Geometry: see drawing. Coordinates: mm, zero at the bounding-box minimum. A direction names the side the tool comes from. Give positions to 0.01 mm unless a question says otherwise; leave off trailing zeros. Write each loop counter-clockwise with the first axis right and the second up, starting at its lowest first coordinate (ties: lowest second). Pieces come first, ordered by that corner, then holes. Notation, with made-up numbers: M 2,27.5 L 16,27.5 A19 cw 16,47.5 Z; hole C 89,29 d1. An arc over 180 degrees is marked long. Use a Markdown table: item, result. Add a question column.
(1) Cut plane B-B (y = 21). Output: boundary loops of the cut face in (x, z).
(2) Material intervals for L1, parallel to Z at x = 5, y = 17; L2, parallel to Y at x = 2.5, z = 15.5; L3, parallel to Z at x = 7, y = 7.5, sorted ascending.
(3) Draft query along Z for the marked faces 4, 5, 6 and 7. Return one class per face: released by +Z, released by -Z, zero draft, split by the parting line, or undercut.
(4) Cut plane A-A (z = 6). Output: boundary loops of the cut face in (x, y).
(5) Cut plane C-C (x = 7.75). Output: boundary loops of the cut face in (y, z).
(6) Pin query (flat end, axial travel): pin 1 Ø1.5 at (x, y) = (9, 9.5) entering from -Z; pin 2 Ø3 at (x, y) = (3, 14) entering from +Z; pin 3 Ø5 at (x, y) = (5, 14) entering from -Z. Return the tip coordinate at first contact, or that it passes through.
(7) Reachability of the marked faces 1, 2 and 3 from +Z, -Z, +X, -X, +Y, -Y: full face, straight path, thin tool, end or side. Return the list, or none.
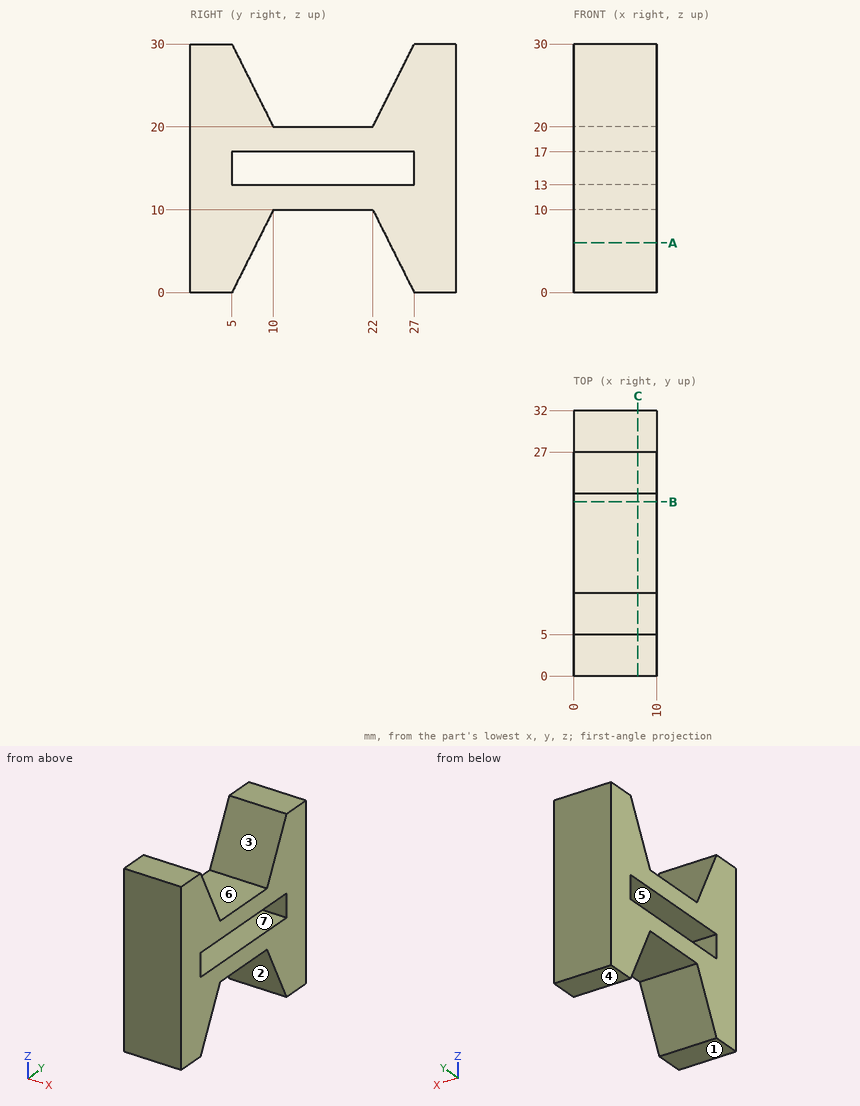
Answer list:
| question | item | result |
|---|---|---|
| 1 | outline | M 0,10 L 10,10 L 10,13 L 0,13 Z; M 0,17 L 10,17 L 10,20 L 0,20 Z |
| 2 | L1 | 10 to 13, 17 to 20 |
| 2 | L2 | 0 to 5, 27 to 32 |
| 2 | L3 | 5 to 13, 17 to 25 |
| 3 | face 4 | released by -Z |
| 3 | face 5 | undercut |
| 3 | face 6 | released by +Z |
| 3 | face 7 | undercut |
| 4 | outline | M 0,0 L 10,0 L 10,8 L 0,8 Z; M 0,24 L 10,24 L 10,32 L 0,32 Z |
| 5 | outline | M 0,0 L 5,0 L 10,10 L 22,10 L 27,0 L 32,0 L 32,30 L 27,30 L 22,20 L 10,20 L 5,30 L 0,30 Z; hole M 5,13 L 27,13 L 27,17 L 5,17 Z |
| 6 | pin 1 | z = 7.5 |
| 6 | pin 2 | z = 20 |
| 6 | pin 3 | z = 10 |
| 7 | face 1 | -Z, +X, -X, +Y, -Y |
| 7 | face 2 | -Z, +X, -X |
| 7 | face 3 | +Z, +X, -X |
